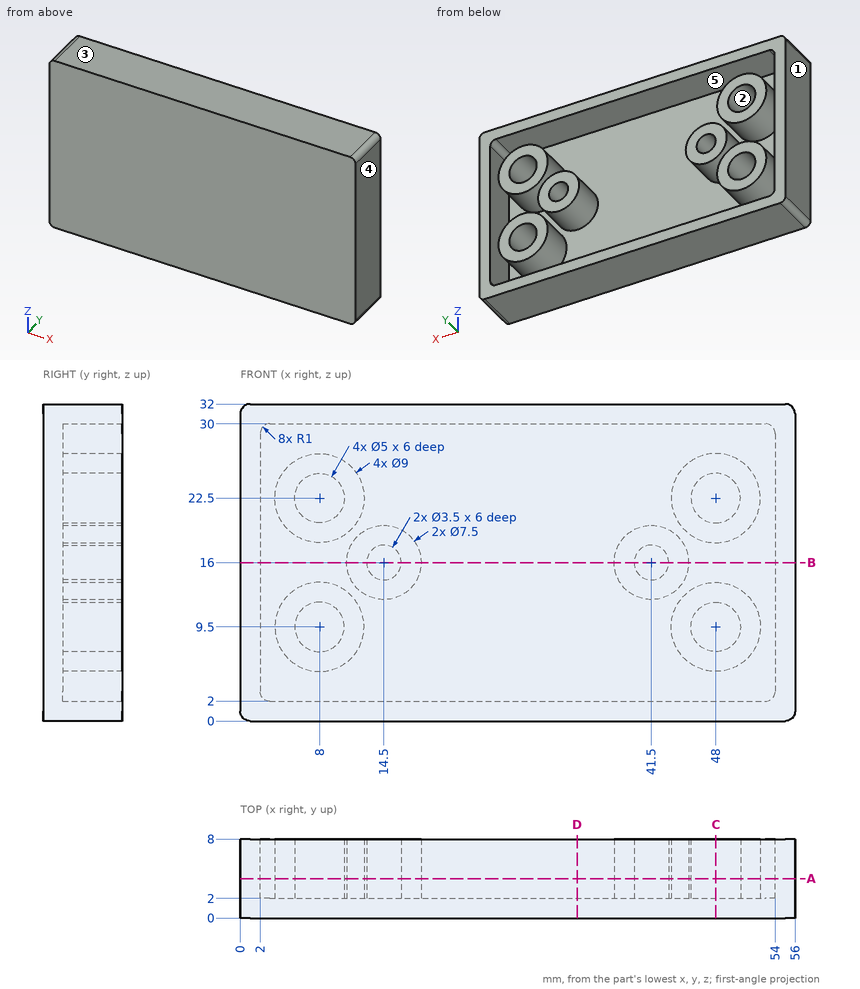
Print and shaded views of the part. All mm, measured from the part's lowest x, y and z. A direction names the side the tool comes from. Coordinates: 2 decimals unless noted, no trailing zeros. Order: outer loops, then holes, each group sorted by start corner. A loop starts at its lowest first (then second) coordinate and runs counter-clockwise, first axis right, second up. Notation, with made-up numbers: (71, 14.5) -> (94, 14.5) arc R27 ccw to (94, 47.5) -> close; hole circle Ø1 at (-25, 41). An arc over 180 degrees is marked (long way). Answer as a JSON object with one key per item and string values. Group by question number.
1) Cut at A-A, the plane y = 4. Count the separate pieces of the cut face and the enclosed holes in it, then the cut area to 3 significant figures.
2) Cut at B-B, the plane z = 16. Write the cut outline in (x, y), then the cut area to 3 significant figures.
3) Which spindle directions (+Z, -Z, +X, -X, +Y, -Y) get a long thin tool onto all of the face, cutting with end or side? Do the marked faces 4 and 5. Say none if no direction does.
4) Pull direction X, two halves, no side cores. Call the marked faces 1, 2 and 3: +X half, -X half, draft (parallel to the pull), parting line (faces both ways), or undercut.
5) Cut at C-C, the plane x = 48. Write the cut outline in (y, z).
6) Cut at D-D, the plane x = 34. Write the cut outline in (y, z).
7) Drill centre lines: L1, parallel to X at y = 5.55, z = 22.5; L2, parallel to X at y = 5.7, z = 16; L3, parallel to X at y = 4.75, z = 4.5. Where is each one in solid material? Low to high.
8) Flat gauge pin, fed straight in: pin 1 (1 mm diameter, centred on x = 15, z = 15.5, fed in from +Y). Where does the tip first touch, or does it go through?
Check values:
{
 "1": {"separate pieces": "7", "enclosed holes": "7", "area": "581 mm²"},
 "2": {"outline": "(0, 0) -> (56, 0) -> (56, 8) -> (54, 8) -> (54, 2) -> (45.25, 2) -> (45.25, 8) -> (43.25, 8) -> (43.25, 2) -> (39.75, 2) -> (39.75, 8) -> (37.75, 8) -> (37.75, 2) -> (18.25, 2) -> (18.25, 8) -> (16.25, 8) -> (16.25, 2) -> (12.75, 2) -> (12.75, 8) -> (10.75, 8) -> (10.75, 2) -> (2, 2) -> (2, 8) -> (0, 8) -> close", "area": "184 mm²"},
 "3": {"face 4": "+Z, -Z, +X, +Y, -Y", "face 5": "+Y"},
 "4": {"face 1": "-X half", "face 2": "undercut", "face 3": "draft"},
 "5": {"outline": "(0, 0) -> (8, 0) -> (8, 2) -> (2, 2) -> (2, 5) -> (8, 5) -> (8, 7) -> (2, 7) -> (2, 12) -> (8, 12) -> (8, 14) -> (2, 14) -> (2, 18) -> (8, 18) -> (8, 20) -> (2, 20) -> (2, 25) -> (8, 25) -> (8, 27) -> (2, 27) -> (2, 30) -> (8, 30) -> (8, 32) -> (0, 32) -> close"},
 "6": {"outline": "(0, 0) -> (8, 0) -> (8, 2) -> (2, 2) -> (2, 30) -> (8, 30) -> (8, 32) -> (0, 32) -> close"},
 "7": {"L1": "x = 0 to 2, 3.5 to 5.5, 10.5 to 12.5, 43.5 to 45.5, 50.5 to 52.5, 54 to 56", "L2": "x = 0 to 2, 10.75 to 12.75, 16.25 to 18.25, 37.75 to 39.75, 43.25 to 45.25, 54 to 56", "L3": "x = 0 to 2, 54 to 56"},
 "8": {"pin 1": "stops at y = 2"}
}
